```python
from build123d import *

# Parameters (mm, degrees)
EXTRUDE_1_DEPTH     = 10
SKETCH_2_R          = 2
CUT_EXTRUDE_1_DEPTH = 84.149305617
SKETCH_3_R          = 1.2
CUT_EXTRUDE_2_DEPTH = 84.149305617


with BuildPart() as part:
    # 草图1 → 凸台-拉伸1 (new body)
    with BuildSketch(Plane.XY):
        with BuildLine():
            Line((-77.394217179, 5), (22.605782821, 5))
            ThreePointArc((22.605782821, 5), (27.605782821, 0), (22.605782821, -5))
            Line((22.605782821, -5), (-77.394217179, -5))
            ThreePointArc((-77.394217179, -5), (-82.394217179, 0), (-77.394217179, 5))
        make_face()
    extrude(amount=EXTRUDE_1_DEPTH)

    # 草图2 → 切除-拉伸1 (cut, through all)
    with BuildSketch(Plane.XY.offset(10)):
        with Locations((-77.394217179, 0)):
            Circle(SKETCH_2_R)
    extrude(amount=-CUT_EXTRUDE_1_DEPTH, mode=Mode.SUBTRACT)

    # 草图3 → 切除-拉伸2 (cut, through all)
    with BuildSketch(Plane.XY.offset(10)):
        with Locations((22.605782821, 0)):
            Circle(SKETCH_3_R)
    extrude(amount=-CUT_EXTRUDE_2_DEPTH, mode=Mode.SUBTRACT)


solid = part.part
```
CAD build for the part. Positions are in the model's coordinates, mm. Round coordinates to 2 decimals unless told otherwise and drop trailing zeros. Write each loop counter-clockwise with the first axis right and the second up, starting at its lowest first coordinate (ties: lowest second). Pieces come first, ordered by that corner, then holes.
Item 1: Band-saw the part on A-A on y = 0. Write the cut outline in (x, z), then the cut area to 3 significant figures.
Filled in:
outline: (-82.39, 0) - (-79.39, 0) - (-79.39, 10) - (-82.39, 10) - close; (-75.39, 0) - (21.41, 0) - (21.41, 10) - (-75.39, 10) - close; (23.81, 0) - (27.61, 0) - (27.61, 10) - (23.81, 10) - close
area: 1,040 mm2
Item 2: Band-saw the part on B-B on z = 3.75. Write the cut outline in (x, y), then the cut area to 3 significant figures.
Filled in:
outline: (-77.39, -5) - (22.61, -5) arc R5 ccw to (22.61, 5) - (-77.39, 5) arc R5 ccw to start; hole circle Ø4 at (-77.39, 0); hole circle Ø2.4 at (22.61, 0)
area: 1,060 mm2
Item 3: Drop flat-ended pins along their axis: pin 1 Ø2 at (y, z) = (-2.5, 3) entering from -X; pin 2 Ø4 at (x, y) = (-2.5, 4) entering from -Z; pin 3 Ø5 at (y, z) = (-3, 1) entering from -X. Give the stop position or say it passes through.
Filled in:
pin 1: stops at x = -82.16
pin 2: stops at z = 0
pin 3: stops at x = -82.37
Item 4: Mould opens along X. For faces 1 (the cylindrical face through (27.605, 0.11, 4.93)), 2 (the flat face through (-27, -5, 5)), 3 (the cylindrical face through (23.714, -0.46, 5.07)) say: released by +X, released by -X, zero draft, split by the parting line, or undercut.
Filled in:
face 1: released by +X
face 2: zero draft
face 3: undercut
Item 5: Drill centre lines: L1, parallel to X at y = -0.75, z = 1.75; L2, parallel to X at y = -4.5, z = 4; L3, parallel to X at y = 1.5, z = 1.5. Where is each one in solid material? Low to high.
Filled in:
L1: x = -82.34 to -79.25, -75.54 to 21.67, 23.54 to 27.55
L2: x = -79.57 to 24.79
L3: x = -82.16 to -78.72, -76.07 to 27.38
